Autodesk Inventor part; units mm, degrees
ref_plane "YZ Plane" through (0, 0, 0) normal (1, 0, 0) x (0, 1, 0)
ref_plane "XZ Plane" through (0, 0, 0) normal (0, 1, 0) x (-1, 0, 0)
ref_plane "XY Plane" through (0, 0, 0) normal (0, 0, 1) x (1, 0, 0)
sketch "Sketch1" plane through (0, 0, 0) normal (0, 0, 1) x (1, 0, 0)
  line L0 (12.065, -7.62) -> (-12.065, -7.62)
  line L1 (-12.065, -7.62) -> (-12.065, 7.62)
  line L2 (-12.065, 7.62) -> (12.065, 7.62)
  line L3 (12.065, 7.62) -> (12.065, -7.62)
  line L4 (12.065, -7.62) -> (-12.065, 7.62) construction
  line L5 (-12.065, -7.62) -> (12.065, 7.62) construction
  point P0 (0, 0)
  dimension "d0" = 24.13
  dimension "d1" = 15.24
extrude "Extrusion1" add sketch "Sketch1" along normal blind 3.175
sketch "Sketch2" plane through (0, 0, 0) normal (0, 0, 1) x (1, 0, 0)
  line L0 (12.065, 7.62) -> (12.065, -7.62)
  line L1 (-12.065, -7.62) -> (-12.065, 7.62)
  line L2 (12.065, -7.62) -> (-12.065, -7.62)
  line L3 (12.065, -7.62) -> (-12.065, -7.62)
  line L4 (-12.065, -7.62) -> (-12.065, -4.445)
  line L5 (-12.065, -4.445) -> (12.065, -4.445)
  line L6 (12.065, -4.445) -> (12.065, -7.62)
  point P0 (0, 0)
  dimension "d4" = 3.175
extrude "Extrusion2" add sketch "Sketch2" against normal blind 12.7
sketch "Sketch3" plane through (-12.065, -4.445, 0) normal (0, 1, 0) x (1, 0, 0)
  line L0 (0, 0) -> (24.13, 0)
  line L1 (12.065, 0) -> (12.065, 12.7) construction
  line L2 (24.13, 12.7) -> (0, 12.7)
  line L3 (24.13, -3.175) -> (0, -3.175)
  point P0 (3.81, 8.382)
  point P1 (20.32, 8.382)
  point P2 (3.81, -6.5118)
  point P3 (20.32, -6.5118)
  dimension "d34" = 16.51
  dimension "d35" = 8.255
  dimension "d37" = 11.557
hole "Hole1" at (-8.255, -4.445, -8.382) at (8.255, -4.445, -8.382) direction (0, -1, 0) diameter 4.191 end through all countersink diameter 7.62 countersink angle 90
sketch "Sketch4" plane through (0, 0, 3.175) normal (0, 0, 1) x (1, 0, 0)
  point P0 (0, 0)
sketch "Sketch5" plane through (0, 0, 3.175) normal (0, 0, 1) x (1, 0, 0)
  line L0 (-12.065, -7.62) -> (12.065, -7.62)
  line L1 (12.065, 7.62) -> (-12.065, 7.62)
  point P0 (0, 0)
  point P1 (0, 4.318)
  dimension "d18" = 11.938
  dimension "d27" = 3.302
hole "Hole2" at (0, 4.318, 3.175) direction (0, 0, -1) diameter 3.7973 end through all
fillet "Fillet2" radius 1.5875 1 edges at (0, -4.445, 0)
fillet "Fillet1" radius 6.35 2 edges at (12.065, 7.62, 1.5875) (-12.065, 7.62, 1.5875)
sketch "Sketch6" plane through (0, 0, 0) normal (0, 0, -1) x (-1, 0, 0)
  circle A0 centre (0, 4.318) radius 1.8986
  line L0 (12.065, -4.445) -> (-12.065, -4.445)
  circle A1 centre (0, 4.699) radius 10.3124
  circle A2 centre (0, 4.318) radius 9.9187 construction
  circle A3 centre (0, 4.318) radius 9.525 construction
  point P0 (0, 0)
  dimension "d38" = 20.6248
  dimension "d39" = 0.381
  dimension "d40" = 19.8374
  dimension "d41" = 19.05
extrude "Extrusion3" cut sketch "Sketch6" along normal up to surface (12.7 mm away)
sketch "Sketch7" plane through (12.065, -4.445, -1.5875) normal (0, 1, 0) x (1, 0, 0)
  circle A0 centre (-20.32, 6.6675) radius 1.2319
  point P0 (-12.065, -1.5875)
properties part number "J005359" material "ALUMINUM, 6061-T651"
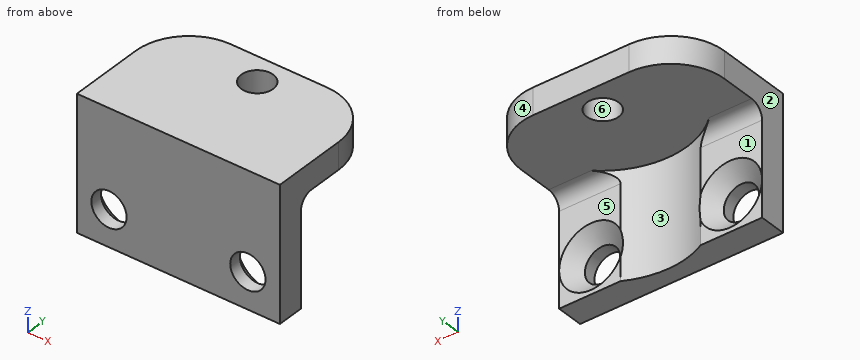
Input: part model. Units: mm. Frame: model coordinates. Face numbers are marked on the shaded views. A direction names the side the tool comes from. Give positions to 0.01 mm unless a question says otherwise; leave off trailing zeros. Order: outer loops, then holes, each group sorted by start corner. A loop starts at its lowest first (then second) coordinate and runs counter-clockwise, first axis right, second up.
Q1. Section C-C on x = -4. Output: boundary loops of the cut face in (y, z) (3 decimals), and give its area (3 significant figures).
Checked values:
outline: (-7.62, -12.7) - (-4.806, -12.7) - (-4.806, 0) - (7.62, 0) - (7.62, 3.175) - (-7.62, 3.175) - close
area: 84.1 mm2
Q2. Contact query for flat-ended pins moving along their axis: pin 1 Ø5 at (x, z) = (8.255, -8.382) entering from +Y (3 decimals); pin 2 Ø3.5 at (x, z) = (7.5, -6) entering from +Y (3 decimals); pin 3 Ø6.5 at (x, y) = (-5.5, 3) entering from -Z; pin 4 Ø3.5 at (x, y) = (0, 4.318) entering from +Z. Output: stop coordinate, or through.
Checked values:
pin 1: stops at y = -5.755
pin 2: stops at y = -4.445
pin 3: stops at z = 0
pin 4: passes through
Q3. Draft query along X for the marked faces 4, 5 and 6. Return one class per face: +X half, -X half, draft (parallel to the pull), parting line (faces both ways), or undercut.
Checked values:
face 4: +X half
face 5: draft
face 6: undercut
Q4. Set-up query: the marked faces 1, 2 and 3. Return all of +Z, -Z, +X, -X, +Y, -Y with unobstructed straight access to the full face (end or side cutting, diameter ignored); none if empty.
Checked values:
face 1: -Z, +X, -X, +Y
face 2: +Z, -Z, -X, +Y, -Y
face 3: -Z, +Y
Q5. Section D-D on z = -9. State how many separate pieces and enclosed holes the cut face has, and give its area (3 significant figures).
Checked values:
separate pieces: 3
enclosed holes: 0
area: 37.6 mm2
Q6. Section B-B on y = 5.75. Output: boundary loops of the cut face in (x, z) (3 decimals), and give its area (3 significant figures).
Checked values:
outline: (-10.215, 0) - (-1.247, 0) - (-1.247, 3.175) - (-10.215, 3.175) - close; (1.247, 0) - (10.215, 0) - (10.215, 3.175) - (1.247, 3.175) - close
area: 57.0 mm2
Q7. Section A-A on x = 0. Output: boundary loops of the cut face in (y, z) (3 decimals).
Checked values:
outline: (-7.62, -12.7) - (-5.613, -12.7) - (-5.613, 0) - (2.419, 0) - (2.419, 3.175) - (-7.62, 3.175) - close; (6.217, 0) - (7.62, 0) - (7.62, 3.175) - (6.217, 3.175) - close
Q8. Ray query, probe 1 along X at (y, z) = (-6.5, -9.5) (3 decimals); probe 2 along Y at (x, z) = (10, -12) (3 decimals); probe 3 along Z at (x, y) = (-0.5, -2.5) (3 decimals). Return the intervals inside material, ascending.
Checked values:
probe 1: x = -12.065 to -10.027, -6.483 to 6.483, 10.027 to 12.065
probe 2: y = -7.62 to -4.445
probe 3: z = 0 to 3.175
